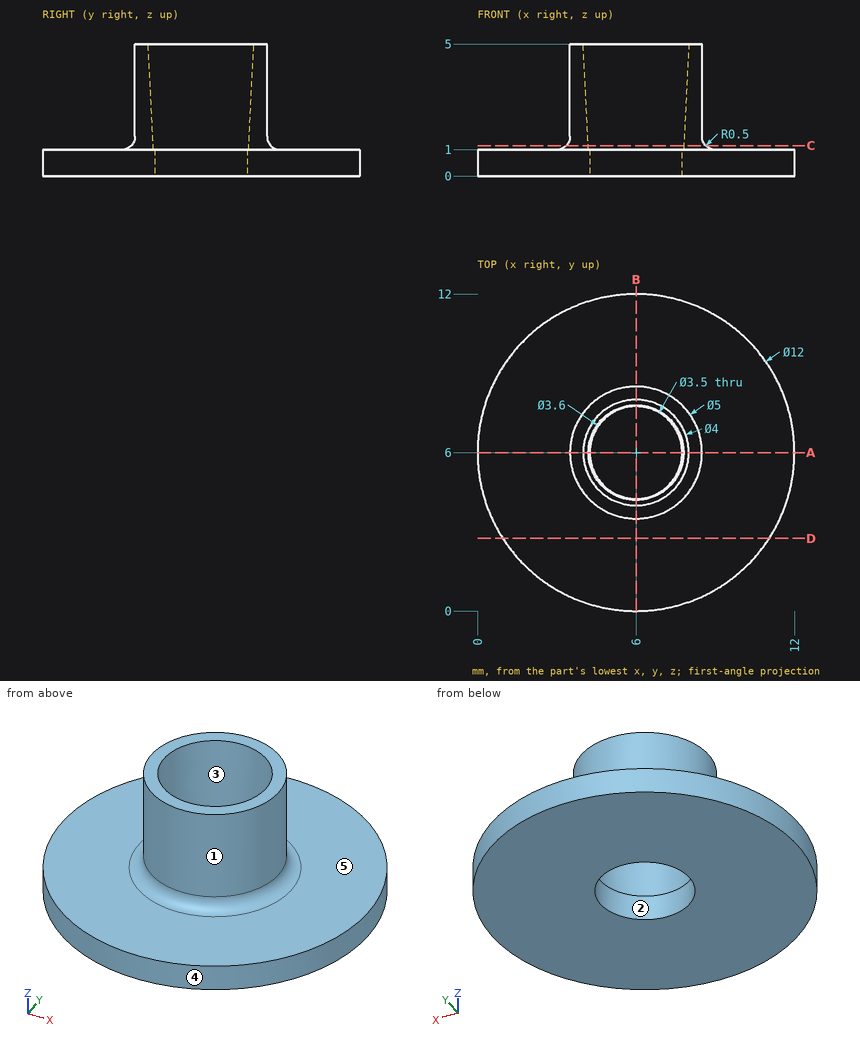
Here's the drawing with two shaded views (mm, measured from the low corner). I have some questions. A direction names the side the tool comes from. Give positions to 0.01 mm unless a question says otherwise; leave off trailing zeros. Order: outer loops, then holes, each group sorted by start corner. A loop starts at its lowest first (then second) coordinate and runs counter-clockwise, first axis right, second up. Notation, with made-up numbers: M -5.75,62 L 45.25,62 A9 ccw 45.25,67 Z; hole C 25,-11 d6. An arc over 180 degrees is marked long. One line per question, with ' | ' between items.
Item 1: Please list where these lines run through material, in increasing order: L1, parallel to Y at x = 6, z = 0.6; L2, parallel to Z at x = 6.25, y = 2.5; L3, parallel to Y at x = 5.25, z = 1.3.
Answer block:
L1: y = 0 to 4.25, 7.75 to 12 | L2: z = 0 to 1 | L3: y = 3.57 to 4.35, 7.65 to 8.43
Item 2: Suppose I cut it at D-D, the plane y = 2.75. Write out the boundary of the cut face in (x, z), then the cut area to 3 significant figures.
Answer block:
outline: M 0.96,0 L 11.04,0 L 11.04,1 L 0.96,1 Z | area: 10.1 mm2
Item 3: We'd pull the mould along Y, two halves only. Please class the marked faces 3, 4 and 5: released by +Y, released by -Y, zero draft, split by the parting line, or undercut.
Answer block:
face 3: undercut | face 4: split by the parting line | face 5: zero draft
Item 4: Suppose I cut it at A-A, the plane y = 6. Write out the boundary of the cut face in (x, z), then the cut area to 3 significant figures.
Answer block:
outline: M 0,0 L 4.25,0 L 4.25,1 L 4.2,1 L 4,5 L 3.5,5 L 3.5,1.5 A0.5 cw 3,1 L 0,1 Z; M 7.75,0 L 12,0 L 12,1 L 9,1 A0.5 cw 8.5,1.5 L 8.5,5 L 8,5 L 7.8,1 L 7.75,1 Z | area: 13.4 mm2
Item 5: Suppose I cut it at C-C, the plane z = 1.15. Write out the boundary of the cut face in (x, y) (1 decimal), then the cut area to 3 significant figures.
Answer block:
outline: C 6,6 d5.3; hole C 6,6 d3.6 | area: 11.7 mm2
Item 6: For the marked faces 1 and 2, which set-ups out of +Z, -Z, +X, -X, +Y, -Y let a thin tool reach every point of the face, with its end or its side?
Answer block:
face 1: +Z | face 2: +Z, -Z
Item 7: I'm going to push flat-ended pins straight in: pin 1 Ø1.5 at (x, z) = (8.5, 1) entering from +Y; pin 2 Ø1 at (x, z) = (4, 3) entering from +Y; pin 3 Ø1.5 at (y, z) = (2, 1) entering from -X. Where does each tip first touch, or does it pass through?
Answer block:
pin 1: stops at y = 11.74 | pin 2: stops at y = 8 | pin 3: stops at x = 0.96
